For this review, take the finished solid that the model builds, in its own axes (mm). A direction names the side the tool comes from. Coordinates: 2 decimals unless noted, no trailing zeros. Write each loop counter-clockwise with the first axis right and the second up, starting at its lowest first coordinate (ties: lowest second). Pieces come first, ordered by that corner, then holes. Notation, with made-up numbers: (-35.5, 56.5) -> (23.5, 56.5) arc R19 ccw to (23.5, 85.5) -> close; hole circle Ø9 at (63, -37). An arc over 180 degrees is marked (long way). Put each result on its own line as item: value. Start each with the question number.
Item 1: Insertion check: P1, Ø1, axis at y = 77.5, z = 1.5, coming from the -X side; P2, Ø1.5, axis at y = 77, z = 8, coming from the -X side; P3, Ø5, axis at y = 85.5, z = 7.5, coming from the +X side; P4, Ø24, axis at x = 35, y = 60, coming from the -Z side. Each pin has a flat end and moves straight along its axis. Give the tip position at first contact, or say it passes through.
Item 2: The part is to be moulded in two halves that separate along X. For faces 1 (the flat face through (0, 30, 5)), 2 (the flat face through (35, 38, 10)), 3 (the cylindrical face through (44.229, 77.743, 4.93)), say which applies: +X half, -X half, draft (parallel to the pull), parting line (faces both ways), or undercut.
Item 3: For faces 4 (the flat face through (35, 15, 5)), 5 (the flat face through (35, 38, 0)), list the 3-axis set-ups (+Z, -Z, +X, -X, +Y, -Y) from which the entire face can be reached by the end or side of a thin tool; tool diameter is ignored.
Item 4: Consider section D-D on x = 59. Give the boundary of the cut face in (y, z).
Item 5: Consider section B-B on y = 47.5. Give the boundary of the cut face in (x, z), and give its area (3 significant figures).
Item 6: Consider section C-C on z = 2. Give the boundary of the cut face in (x, y).
Item 7: To check wall thickness, follow L1, parallel to Y at x = 35, z = 5.25; L2, parallel to Y at x = 20, z = 2; L3, parallel to Y at x = 56, z = 6.25. State the ranges of each line that lie inside material, in increasing order.
Item 8: Consider section A-A on x = 35. Give the boundary of the cut face in (y, z).
Autodesk Fusion 360 part; units mm, degrees
sketch "Sketch1" plane through (0, 0, 0) normal (0, 0, 1) x (1, 0, 0)
  line L0 (0, 0) -> (70, 0)
  line L1 (70, 0) -> (70, 60)
  line L2 (0, 60) -> (0, 0)
  arc A0 (70, 60) -> (0, 60) centre (35, 60) ccw
  circle A1 centre (35, 60) radius 20
  line L3 (10, 30) -> (60, 30)
  line L4 (60, 30) -> (60, 15)
  line L5 (60, 15) -> (10, 15)
  line L6 (10, 15) -> (10, 30)
  dimension "d1" = 70
  dimension "d2" = 60
  dimension "d3" = 40
  dimension "d4" = 50
  dimension "d5" = 15
  dimension "d6" = 10
  dimension "d7" = 15
extrude "Extrude1" add sketch "Sketch1" along normal blind 10
Return value:
1. P1: x = 4.41
1. P2: x = 4
1. P3: x = 61.38
1. P4: through
2. face 1: -X half
2. face 2: draft
2. face 3: undercut
3. face 4: +Z, -Z
3. face 5: -Z, +X, -X, +Y, -Y
4. outline: (0, 0) -> (15, 0) -> (15, 10) -> (0, 10) -> close; (30, 0) -> (85.48, 0) -> (85.48, 10) -> (30, 10) -> close
5. outline: (0, 0) -> (19.39, 0) -> (19.39, 10) -> (0, 10) -> close; (50.61, 0) -> (70, 0) -> (70, 10) -> (50.61, 10) -> close
5. area: 388 mm^2
6. outline: (0, 0) -> (70, 0) -> (70, 60) arc R35 ccw to (0, 60) -> close; hole (10, 15) -> (60, 15) -> (60, 30) -> (10, 30) -> close; hole circle Ø40 at (35, 60)
7. L1: 0 to 15, 30 to 40, 80 to 95
7. L2: 0 to 15, 30 to 46.77, 73.23 to 91.62
7. L3: 0 to 15, 30 to 88
8. outline: (0, 0) -> (15, 0) -> (15, 10) -> (0, 10) -> close; (30, 0) -> (40, 0) -> (40, 10) -> (30, 10) -> close; (80, 0) -> (95, 0) -> (95, 10) -> (80, 10) -> close
